Drawing for the job (mm, zero at the part's lowest x, y, z). A direction names the side the tool comes from. Give positions to 0.01 mm unless a question says otherwise; leave off trailing zeros. Order: outer loops, then holes, each group sorted by start corner. A loop starts at its lowest first (then second) coordinate and runs counter-clockwise, first axis right, second up. Notation, with made-up numbers: (10.5, 34.5) - (45.5, 34.5) arc R6 cw to (45.5, 45.5) - close; hole circle Ø6 at (89.5, 69.5). An arc over 180 degrees is marked (long way). One line per item, written item: value.
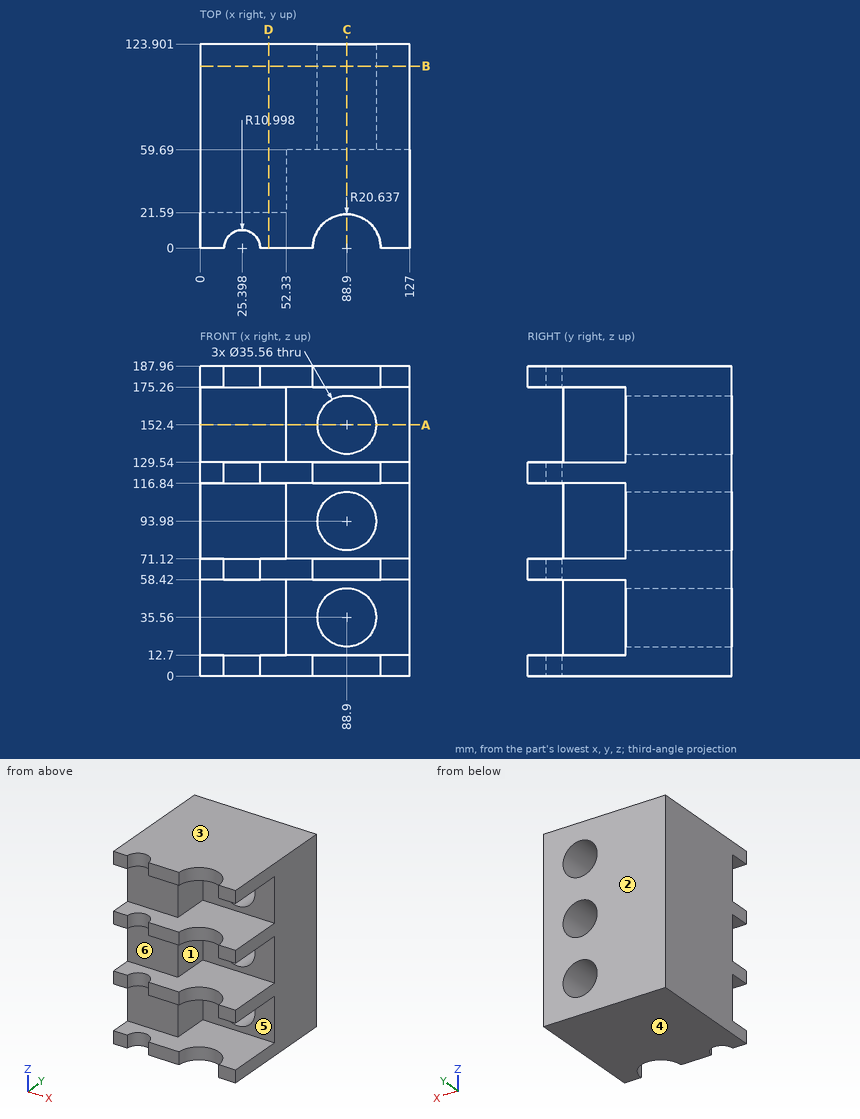
1) Mould opens along Z. For the marked faces 1, 2 and 3 say: released by +Z, released by -Z, zero draft, split by the parting line, or undercut.
Outcome:
face 1: undercut
face 2: zero draft
face 3: released by +Z
2) Cut at B-B, the plane y = 110.5. Give the cut face in (x, z), then the cut area to 3 significant figures.
Outcome:
outline: (0, 0) - (127, 0) - (127, 187.96) - (0, 187.96) - close; hole circle Ø35.56 at (88.9, 35.56); hole circle Ø35.56 at (88.9, 93.98); hole circle Ø35.56 at (88.9, 152.4)
area: 20,900 mm^2
3) Cut at A-A, the plane z = 152.4. Give the cut face in (x, y).
Outcome:
outline: (0, 21.59) - (52.33, 21.59) - (52.33, 59.69) - (71.12, 59.69) - (71.12, 123.9) - (0, 123.9) - close; (106.68, 59.69) - (127, 59.69) - (127, 123.9) - (106.68, 123.9) - close
4) Cut at D-D, the plane x = 41.5. Give the cut face in (y, z).
Outcome:
outline: (0, 0) - (123.9, 0) - (123.9, 187.96) - (0, 187.96) - (0, 175.26) - (21.59, 175.26) - (21.59, 129.54) - (0, 129.54) - (0, 116.84) - (21.59, 116.84) - (21.59, 71.12) - (0, 71.12) - (0, 58.42) - (21.59, 58.42) - (21.59, 12.7) - (0, 12.7) - close
5) Cut at C-C, the plane x = 88.9. Give the cut face in (y, z).
Outcome:
outline: (20.64, 0) - (123.9, 0) - (123.9, 17.78) - (59.69, 17.78) - (59.69, 12.7) - (20.64, 12.7) - close; (20.64, 58.42) - (59.69, 58.42) - (59.69, 53.34) - (123.9, 53.34) - (123.9, 76.2) - (59.69, 76.2) - (59.69, 71.12) - (20.64, 71.12) - close; (20.64, 116.84) - (59.69, 116.84) - (59.69, 111.76) - (123.9, 111.76) - (123.9, 134.62) - (59.69, 134.62) - (59.69, 129.54) - (20.64, 129.54) - close; (20.64, 175.26) - (59.69, 175.26) - (59.69, 170.18) - (123.9, 170.18) - (123.9, 187.96) - (20.64, 187.96) - close
6) Pin check, flat tips, straight feed: pin 1 (13.5 mm diameter, centred on x = 39, z = 40, fed in from -Y); pin 2 (1 mm diameter, centred on x = 82.5, z = 122, fed in from -Y); pin 3 (11.5 mm diameter, centred on y = 33, z = 28, fed in from +X). Stop position of each tip, or through.
Outcome:
pin 1: stops at y = 21.59
pin 2: stops at y = 19.45
pin 3: stops at x = 52.33
7) Drill centre lines: line 1 along Z through (x, y) = (72.5, 59.5); line 2 along X through (y, z) = (94.5, 35.56); line 3 along Y through (x, z) = (42, 132). Where is each one in solid material? Low to high. Write a range as from..to.
Outcome:
line 1: z = 0..12.7, 58.42..71.12, 116.84..129.54, 175.26..187.96
line 2: x = 0..71.12, 106.68..127
line 3: y = 21.59..123.9
8) Which spindle directions (+Z, -Z, +X, -X, +Y, -Y) get a long thin tool onto all of the face, cutting with end or side? Do the marked faces 4, 5 and 6. Say none if no direction does.
Outcome:
face 4: -Z, +X, -X, +Y, -Y
face 5: +X, -Y
face 6: +X, -X, -Y
